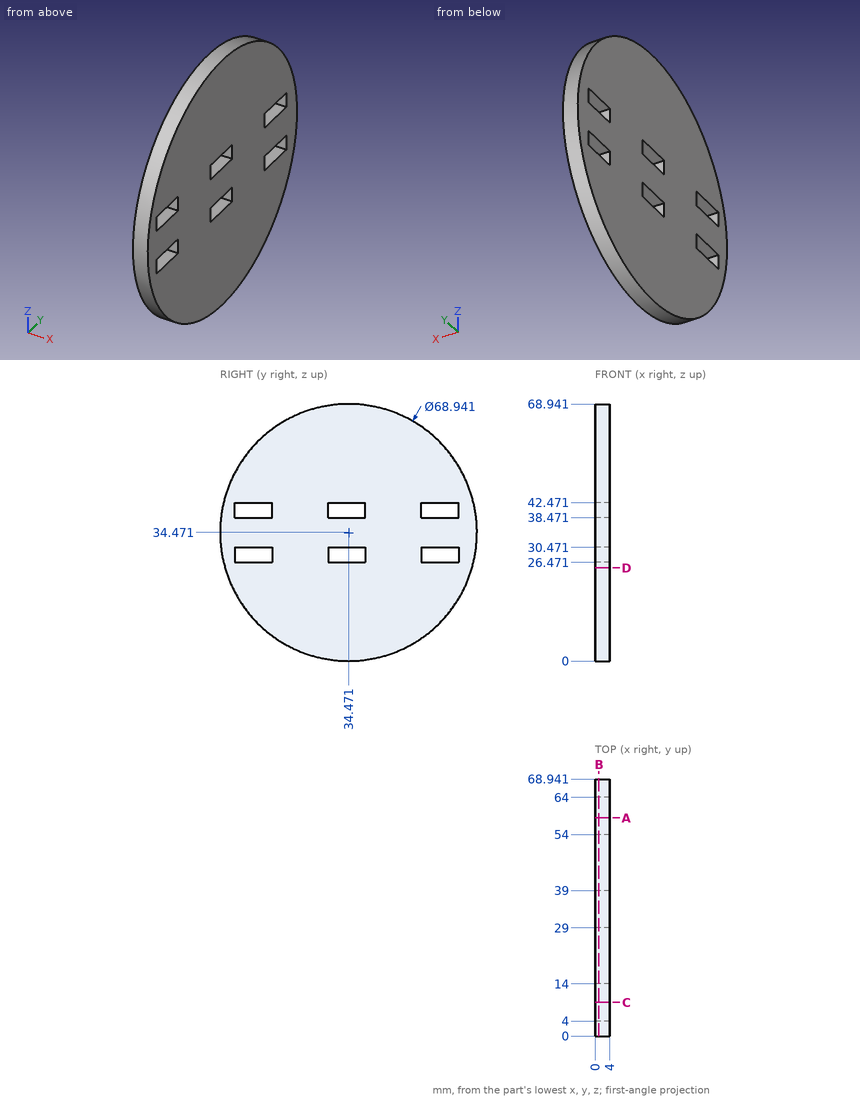
Could you check a few things on this drawing? It's one solid part, dimensions in mm from its lowest x, y, z. Coordinates: 2 decimals unless noted, no trailing zeros. Loops run counter-clockwise (first coordinate to the right, second up) from the corner with the lowest first, then second, coordinate; pieces in that order, holes last.
1. Imagine slicing it at C-C (y = 9). Please give me the cut outline in (x, z), and give its area (3 significant figures).
2. Imagine slicing it at B-B (x = 1.05). Please give me the cut outline in (y, z).
3. I need wall thicknesses on L1, parallel to Z at x = 2.4, y = 62 (1 decimal); L2, parallel to Z at x = 0.5, y = 58.5 (1 decimal); L3, parallel to Y at x = 0.65, z = 28. Which ranges of each line are inside material? Lowest first, please.
4. For P1, Ø4, axis at y = 35.5, z = 50, coming from the -X side; P2, Ø2, axis at x = 2, y = 61, coming from the +Z side; P3, Ø2, axis at x = 1.5, z = 41, coming from the -Y side; P4, Ø1.2, axis at x = 3, z = 29, coming from the -Y side, each with a flat end and sliding along its axis, tell me the tip position at first contact or that it passes through.
5. Imagine slicing it at A-A (y = 58.5). Please give me the cut outline in (x, z) (1 decimal), and give its area (3 significant figures).
6. Imagine slicing it at D-D (z = 25). Please give me the cut outline in (x, y) (1 decimal), and give its area (3 significant figures).
Computed values:
1. outline: (0, 11.24) - (4, 11.24) - (4, 26.47) - (0, 26.47) - close; (0, 30.47) - (4, 30.47) - (4, 38.47) - (0, 38.47) - close; (0, 42.47) - (4, 42.47) - (4, 57.7) - (0, 57.7) - close
1. area: 154 mm2
2. outline: circle Ø68.94 at (34.47, 34.47); hole (4, 26.47) - (14, 26.47) - (14, 30.47) - (4, 30.47) - close; hole (4, 38.47) - (14, 38.47) - (14, 42.47) - (4, 42.47) - close; hole (29, 26.47) - (39, 26.47) - (39, 30.47) - (29, 30.47) - close; hole (29, 38.47) - (39, 38.47) - (39, 42.47) - (29, 42.47) - close; hole (54, 26.47) - (64, 26.47) - (64, 30.47) - (54, 30.47) - close; hole (54, 38.47) - (64, 38.47) - (64, 42.47) - (54, 42.47) - close
3. L1: z = 13.7 to 26.5, 30.5 to 38.5, 42.5 to 55.2
3. L2: z = 9.8 to 26.5, 30.5 to 38.5, 42.5 to 59.2
3. L3: y = 0.61 to 4, 14 to 29, 39 to 54, 64 to 68.33
4. P1: stops at x = 0
4. P2: stops at z = 57.63
4. P3: stops at y = 0.45
4. P4: stops at y = 0.35
5. outline: (0, 9.8) - (4, 9.8) - (4, 26.5) - (0, 26.5) - close; (0, 30.5) - (4, 30.5) - (4, 38.5) - (0, 38.5) - close; (0, 42.5) - (4, 42.5) - (4, 59.2) - (0, 59.2) - close
5. area: 166 mm2
6. outline: (0, 1.3) - (4, 1.3) - (4, 67.6) - (0, 67.6) - close
6. area: 265 mm2
